from build123d import *

# Parameters (mm, degrees)
SKETCH_1_W                         = 127
SKETCH_1_H                         = 73
SKETCH_1_R                         = 5
SM_BASE_FLANGE_1_DEPTH             = 3
SM_EDGE_FLANGE_1_STRIP_W           = 13.48
SM_EDGE_FLANGE_1_STRIP_H           = 3
SM_EDGE_FLANGE_1_STRIP_CUT_DEPTH   = 127
SM_EDGE_FLANGE_1_STRIP_2_W         = 13.48
SM_EDGE_FLANGE_1_STRIP_2_H         = 3
SM_EDGE_FLANGE_1_STRIP_CUT_2_DEPTH = 127
SM_EDGE_FLANGE_1_DEPTH             = 127
SM_EDGE_FLANGE_1_BEND_DEPTH        = 127
SKETCH_12_OUTSIDE_W                = 159.708
SKETCH_12_OUTSIDE_H                = 78.708
SKETCH_12_OUTSIDE_R                = 5
CUT_EXTRUDE_4_DEPTH                = 108.131928014
SM_EDGE_FLANGE_2_STRIP_W           = 13.48
SM_EDGE_FLANGE_2_STRIP_H           = 3
SM_EDGE_FLANGE_2_STRIP_CUT_DEPTH   = 65.52
SM_EDGE_FLANGE_2_STRIP_2_W         = 13.48
SM_EDGE_FLANGE_2_STRIP_2_H         = 3
SM_EDGE_FLANGE_2_STRIP_CUT_2_DEPTH = 65.52
SM_EDGE_FLANGE_2_DEPTH             = 65.52
SM_START                           = 3
SM_EDGE_FLANGE_2_PROFILE_W         = 65.52
SM_EDGE_FLANGE_2_PROFILE_H         = 19.26
SM_EDGE_FLANGE_2_PROFILE_R         = 5
SM_EDGE_FLANGE_2_FLAT_DEPTH        = 3
SM_EDGE_FLANGE_2_BEND_DEPTH        = 65.52
SM_EDGE_FLANGE_2_PROFILE_2_W       = 65.52
SM_EDGE_FLANGE_2_PROFILE_2_H       = 19.26
SM_EDGE_FLANGE_2_PROFILE_2_R       = 5
SM_EDGE_FLANGE_2_FLAT_2_DEPTH      = 3


# Sheet-metal steps are written as plain solids
with BuildPart() as part:
    # Sketch 1 → Базовая кромка1 (new body)
    with BuildSketch(Plane.XY):
        Rectangle(SKETCH_1_W, SKETCH_1_H)
        with Locations((-54.25, 0)):
            Circle(SKETCH_1_R, mode=Mode.SUBTRACT)
        with Locations((54.25, 0)):
            Circle(SKETCH_1_R, mode=Mode.SUBTRACT)
    extrude(amount=-SM_BASE_FLANGE_1_DEPTH)

    # Ребро-кромка1 strip (across the edge) → Ребро-кромка1 strip cut (cut)
    with BuildSketch(Plane(origin=(-63.5, 36.5, -3), x_dir=(0, -1, 0), z_dir=(1, 0, 0))):
        with Locations((-3, -1.5)):
            Rectangle(SM_EDGE_FLANGE_1_STRIP_W, SM_EDGE_FLANGE_1_STRIP_H)
    extrude(amount=SM_EDGE_FLANGE_1_STRIP_CUT_DEPTH, mode=Mode.SUBTRACT)

    # Ребро-кромка1 strip 2 (across the edge) → Ребро-кромка1 strip cut 2 (cut)
    with BuildSketch(Plane(origin=(63.5, -36.5, -3), x_dir=(0, 1, 0), z_dir=(-1, 0, 0))):
        with Locations((-3, -1.5)):
            Rectangle(SM_EDGE_FLANGE_1_STRIP_2_W, SM_EDGE_FLANGE_1_STRIP_2_H)
    extrude(amount=SM_EDGE_FLANGE_1_STRIP_CUT_2_DEPTH, mode=Mode.SUBTRACT)

    # Ребро-кромка1 section (across the edge) → Ребро-кромка1 (add)
    with BuildSketch(Plane(origin=(-63.5, 36.5, -3), x_dir=(0, -1, 0), z_dir=(1, 0, 0))):
        with BuildLine():
            Line((0, 0.74), (0, 43))
            Line((0, 43), (3, 43))
            Line((3, 43), (3, 0.74))
            ThreePointArc((3, 0.74), (3.216740982, 0.216740982), (3.74, 0))
            Line((3.74, 0), (3.74, -3))
            ThreePointArc((3.74, -3), (1.095420638, -1.904579362), (0, 0.74))
        make_face()
    extrude(amount=SM_EDGE_FLANGE_1_DEPTH)

    # Ребро-кромка1 section 2 (across the edge) → Ребро-кромка1 bend (add)
    with BuildSketch(Plane(origin=(63.5, -36.5, -3), x_dir=(0, 1, 0), z_dir=(-1, 0, 0))):
        with BuildLine():
            Line((0, 0.74), (0, 43))
            Line((0, 43), (3, 43))
            Line((3, 43), (3, 0.74))
            ThreePointArc((3, 0.74), (3.216740982, 0.216740982), (3.74, 0))
            Line((3.74, 0), (3.74, -3))
            ThreePointArc((3.74, -3), (1.095420638, -1.904579362), (0, 0.74))
        make_face()
    extrude(amount=SM_EDGE_FLANGE_1_BEND_DEPTH)

    # Эскиз12 outside → Вырез-Вытянуть4 (cut, through all)
    # profile 1 of 3: a face of its own
    with BuildSketch(Plane(origin=(0, 36.5, 0), x_dir=(1, 0, 0), z_dir=(0, 1, 0))):
        with Locations((0, 23)):
            Rectangle(SKETCH_12_OUTSIDE_W, SKETCH_12_OUTSIDE_H)
        with BuildLine():
            Line((63.5, 14), (49.900936783, 40.557776255))
            ThreePointArc((49.900936783, 40.557776255), (38.655790946, 45.721351959), (31, 36))
            Line((31, 36), (31, 24))
            Line((31, 24), (-31, 24))
            Line((-31, 24), (-31, 36))
            ThreePointArc((-31, 36), (-38.655790946, 45.721351959), (-49.900936783, 40.557776255))
            Line((-49.900936783, 40.557776255), (-63.5, 14))
            Line((-63.5, 14), (-63.5, 0))
            Line((-63.5, 0), (-38.5, 0))
            Line((-38.5, 0), (-38.5, 5))
            Line((-38.5, 5), (38.5, 5))
            Line((38.5, 5), (38.5, 0))
            Line((38.5, 0), (63.5, 0))
            Line((63.5, 0), (63.5, 14))
        make_face(mode=Mode.SUBTRACT)
    # profile 2 of 3: a face of its own
    with BuildSketch(Plane(origin=(0, 36.5, 0), x_dir=(1, 0, 0), z_dir=(0, 1, 0))):
        with Locations(Location((41, 36, 0), (0, 0, 270))):
            Circle(SKETCH_12_OUTSIDE_R)
    # profile 3 of 3: a face of its own
    with BuildSketch(Plane(origin=(0, 36.5, 0), x_dir=(1, 0, 0), z_dir=(0, 1, 0))):
        with Locations(Location((-41, 36, 0), (0, 0, 270))):
            Circle(SKETCH_12_OUTSIDE_R)
    extrude(amount=-CUT_EXTRUDE_4_DEPTH, mode=Mode.SUBTRACT)

    # Ребро-кромка2 strip (across the edge) → Ребро-кромка2 strip cut (cut)
    with BuildSketch(Plane(origin=(38.5, -32.76, -3), x_dir=(1, 0, 0), z_dir=(0, 1, 0))):
        with Locations((-6, -1.5)):
            Rectangle(SM_EDGE_FLANGE_2_STRIP_W, SM_EDGE_FLANGE_2_STRIP_H)
    extrude(amount=SM_EDGE_FLANGE_2_STRIP_CUT_DEPTH, mode=Mode.SUBTRACT)

    # Ребро-кромка2 strip 2 (across the edge) → Ребро-кромка2 strip cut 2 (cut)
    with BuildSketch(Plane(origin=(-38.5, 32.76, -3), x_dir=(-1, 0, 0), z_dir=(0, -1, 0))):
        with Locations((-6, -1.5)):
            Rectangle(SM_EDGE_FLANGE_2_STRIP_2_W, SM_EDGE_FLANGE_2_STRIP_2_H)
    extrude(amount=SM_EDGE_FLANGE_2_STRIP_CUT_2_DEPTH, mode=Mode.SUBTRACT)

    # Ребро-кромка2 bend section (across the edge) → Ребро-кромка2 (add)
    with BuildSketch(Plane(origin=(38.5, -32.76, -3), x_dir=(1, 0, 0), z_dir=(0, 1, 0))):
        with BuildLine():
            Line((-3, 0.74), (0, 0.74))
            ThreePointArc((0, 0.74), (0.216740982, 0.216740982), (0.74, 0))
            Line((0.74, 0), (0.74, -3))
            ThreePointArc((0.74, -3), (-1.904579362, -1.904579362), (-3, 0.74))
        make_face()
    extrude(amount=SM_EDGE_FLANGE_2_DEPTH)

    # Ребро-кромка2 profile (on flange) → Ребро-кромка2 flat (add)
    with BuildSketch(Plane(origin=(38.5, 0, -3), x_dir=(0, 1, 0), z_dir=(-1, 0, 0)).offset(SM_START)):
        with Locations((0, 10.37)):
            Rectangle(SM_EDGE_FLANGE_2_PROFILE_W, SM_EDGE_FLANGE_2_PROFILE_H)
        with Locations((22.031313941, 10)):
            Circle(SM_EDGE_FLANGE_2_PROFILE_R, mode=Mode.SUBTRACT)
        with Locations((-22.031313941, 10)):
            Circle(SM_EDGE_FLANGE_2_PROFILE_R, mode=Mode.SUBTRACT)
    extrude(amount=-SM_EDGE_FLANGE_2_FLAT_DEPTH)

    # Ребро-кромка2 bend section 2 (across the edge) → Ребро-кромка2 bend (add)
    with BuildSketch(Plane(origin=(-38.5, 32.76, -3), x_dir=(-1, 0, 0), z_dir=(0, -1, 0))):
        with BuildLine():
            Line((-3, 0.74), (0, 0.74))
            ThreePointArc((0, 0.74), (0.216740982, 0.216740982), (0.74, 0))
            Line((0.74, 0), (0.74, -3))
            ThreePointArc((0.74, -3), (-1.904579362, -1.904579362), (-3, 0.74))
        make_face()
    extrude(amount=SM_EDGE_FLANGE_2_BEND_DEPTH)

    # Ребро-кромка2 profile 2 (on flange) → Ребро-кромка2 flat 2 (add)
    with BuildSketch(Plane(origin=(-38.5, 0, -3), x_dir=(0, -1, 0), z_dir=(1, 0, 0)).offset(SM_START)):
        with Locations((0, 10.37)):
            Rectangle(SM_EDGE_FLANGE_2_PROFILE_2_W, SM_EDGE_FLANGE_2_PROFILE_2_H)
        with Locations((-22.031313941, 10)):
            Circle(SM_EDGE_FLANGE_2_PROFILE_2_R, mode=Mode.SUBTRACT)
        with Locations((22.031313941, 10)):
            Circle(SM_EDGE_FLANGE_2_PROFILE_2_R, mode=Mode.SUBTRACT)
    extrude(amount=-SM_EDGE_FLANGE_2_FLAT_2_DEPTH)


solid = part.part
Build history of the part. All positions in model axes, mm. A direction names the side the tool comes from. Round coordinates to 2 decimals unless told otherwise and drop trailing zeros. Write each loop counter-clockwise with the first axis right and the second up, starting at its lowest first coordinate (ties: lowest second). Pieces come first, ordered by that corner, then holes. Notation, with made-up numbers: M -35,-35.75 L 11,-35.75 A7 ccw 11,-22.75 Z; hole C 39.25,-16 d5. An arc over 180 degrees is marked long. Use CSV: the item, a comma, the result in double quotes.
1. Saw through at D-D (x = -12). Give the cut face in (y, z).
Reply:
outline,"M -36.5,-24 L -33.5,-24 L -33.5,-5 L -36.5,-5 Z; M 33.5,-24 L 36.5,-24 L 36.5,-5 L 33.5,-5 Z"
2. Saw through at A-A (x = -41). Give the cut face in (y, z).
Reply:
outline,"M -36.5,-46 L -33.5,-46 L -33.5,-41 L -36.5,-41 Z; M -36.5,-31 L -33.5,-31 L -33.5,-3.74 A0.74 cw -32.76,-3 L 32.76,-3 A0.74 cw 33.5,-3.74 L 33.5,-31 L 36.5,-31 L 36.5,-3.74 A3.74 ccw 32.76,0 L -32.76,0 A3.74 ccw -36.5,-3.74 Z; M 33.5,-46 L 36.5,-46 L 36.5,-41 L 33.5,-41 Z"
3. Wall check: probe 1 along Y at (x, z) = (36.8, -13); probe 2 along Y at (x, z) = (-37, -22); probe 3 along Y at (x, z) = (-19.5, -9). Give the ranges that are in metal, low to high. Write a range as from..to.
Reply:
probe 1,"y = -36.5..-33.5, -32.76..-27.03, -17.03..17.03, 27.03..32.76, 33.5..36.5"
probe 2,"y = -36.5..-33.5, -32.76..32.76, 33.5..36.5"
probe 3,"y = -36.5..-33.5, 33.5..36.5"
4. Saw through at C-C (z = -26). Give the cut face in (x, y).
Reply:
outline,"M -57.36,-36.5 L -31,-36.5 L -31,-33.5 L -57.36,-33.5 Z; M -57.36,33.5 L -31,33.5 L -31,36.5 L -57.36,36.5 Z; M 31,-36.5 L 57.36,-36.5 L 57.36,-33.5 L 31,-33.5 Z; M 31,33.5 L 57.36,33.5 L 57.36,36.5 L 31,36.5 Z"
5. Two-plate mould, pull along Y, no slides. Class faces 1 (the face through (-50.82, -35.38, -1.07)), 2 (the face through (-37, 32.76, -11)), 3 (the face through (-38.5, 35, -2)): +Y half, -Y half, draft (parallel to the pull), parting line (faces both ways), or undercut.
Reply:
face 1,"-Y half"
face 2,"undercut"
face 3,"draft"
6. Flat gauge pins, fed straight in: pin 1 (6 mm diameter, centred on y = -15, z = -18.5, fed in from +X); pin 2 (16 mm diameter, centred on x = -54.25, y = 0, fed in from -Z); pin 3 (16 mm diameter, centred on y = 22.03, z = -13, fed in from -X). Where does each tip first touch, or does it go through?
Reply:
pin 1,"stops at x = 38.5"
pin 2,"stops at z = -3"
pin 3,"stops at x = -38.5"
7. Tool access for faces 4 (the face through (-36.62, 0.46, -1.07)), 5 (the face through (-35.5, 0, -14)), 6 (the face through (-1, 33.5, -16)): list every direction of +Z, -Z, +X, -X, +Y, -Y with a clear straight run to the whole face (end or side of a thin tool).
Reply:
face 4,"+Z, +Y, -Y"
face 5,"+Z, -Z"
face 6,"-Z, +X, -X"
8. Saw through at B-B (y = 30.5). Give the cut face in (x, z), plus the area to 3 significant figures.
Reply:
outline,"M -63.5,-3 L -39.24,-3 A0.74 cw -38.5,-3.74 L -38.5,-23 L -35.5,-23 L -35.5,-3.74 A3.74 ccw -39.24,0 L -63.5,0 Z; M 35.5,-23 L 38.5,-23 L 38.5,-3.74 A0.74 cw 39.24,-3 L 63.5,-3 L 63.5,0 L 39.24,0 A3.74 ccw 35.5,-3.74 Z"
area,"282 mm²"
